Part model, mm, in its own coordinate system. A direction names the side the tool comes from. Coordinates: 2 decimals unless noted, no trailing zeros. Order: outer loops, then holes, each group sorted by start corner. A loop starts at its lowest first (then second) coordinate and runs counter-clockwise, first axis right, second up. Notation, with made-up numbers: (18, 46.5) - (70, 46.5) arc R18 ccw to (70, 55.5) - close; hole circle Ø5 at (50, 44). An arc over 180 degrees is marked (long way). Use a Markdown table: item, result. Add a question column.
1) Two-plate mould, pull along X, no slides. Class faces 1 (the face through (6, 14, 51)), 2 (the face through (11, 5.8, 44)), 3 (the face through (11, 16.3, 44)), 4 (the face through (10, 5, 0)): +X half, -X half, draft (parallel to the pull), parting line (faces both ways), or undercut.
2) Tool access for faces 5 (the face through (11, 20, 80)), 6 (the face through (7, 8.3, 44)), 7 (the face through (10, 17, 0)), 8 (the face through (15, 6, 44)): list every direction of +Z, -Z, +X, -X, +Y, -Y with a clear straight run to the whole face (end or side of a thin tool).
3) Saw through at B-B on x = 14. List the corners of the cut face in (y, z), then the cut area to 3 significant figures.
4) Wall check: L1, parallel to Y at x = 8.75, z = 13; L2, parallel to Y at x = 11.25, z = 56; L3, parallel to Z at x = 15, y = 9.25. Give the ranges that are in metal, low to high. Write a range as [from, to].
5) Saw through at A-A on z = 31. List the corners of the cut face in (x, y).
6) Drop flat-ended pins along their axis: P1, Ø1.1, axis at x = 14, z = 64.5, coming from the +Y side; P2, Ø1.3, axis at y = 7, z = 53, coming from the +X side; P3, Ø3, axis at x = 14, y = 11, coming from the -Z side; P4, Ø1, axis at y = 11.5, z = 22, coming from the -X side. Give the stop position or say it passes through.
7) Saw through at D-D on x = 10. List the corners of the cut face in (y, z), then the cut area to 3 significant figures.
8) Saw through at C-C on y = 19.75. List the corners of the cut face in (x, z), then the cut area to 3 significant figures.
```python
from build123d import *

# Parameters (mm, degrees)
SKETCH2_W           = 3.75
SKETCH2_H           = 0.3
SKETCH2_H_2         = 0.2
BOSS_EXTRUDE3_DEPTH = 90
SKETCH3_W           = 10.75
SKETCH3_H           = 15.726491146
BOSS_EXTRUDE4_DEPTH = 10
SKETCH4_W           = 10.75
SKETCH4_H           = 2.578461227
BOSS_EXTRUDE5_DEPTH = 20


with BuildPart() as part:
    # Sketch2 → Boss-Extrude3 (new body)
    with BuildSketch(Plane.XY):
        with Locations((14.875, 16.15)):
            Rectangle(SKETCH2_W, SKETCH2_H)
        Polygon((8.7, 16.3), (8.7, 18.913245573), (16.75, 18.913245573), (16.75, 16.3), (13, 16.3), align=None)
        Polygon((6, 18.913245573), (6, 13.8), (8.7, 13.8), (8.7, 16.3), (8.7, 18.913245573), align=None)
        Polygon((8.8, 3.186754427), (8.8, 5.8), (8.8, 8.3), (6, 8.3), (6, 3.186754427), align=None)
        Polygon((8.8, 5.8), (13, 5.8), (16.75, 5.8), (16.75, 3.186754427), (8.8, 3.186754427), align=None)
        with Locations((14.875, 5.9)):
            Rectangle(SKETCH2_W, SKETCH2_H_2)
    extrude(amount=BOSS_EXTRUDE3_DEPTH)

    # Sketch3 → Boss-Extrude4 (add)
    with BuildSketch(Plane.XY.offset(90)):
        with Locations((11.375, 11.05)):
            Rectangle(SKETCH3_W, SKETCH3_H)
    extrude(amount=BOSS_EXTRUDE4_DEPTH)

    # Sketch4 → Boss-Extrude5 (add)
    with BuildSketch(Plane.XY.offset(100)):
        with Locations((11.375, 20.202476187)):
            Rectangle(SKETCH4_W, SKETCH4_H)
    extrude(amount=-BOSS_EXTRUDE5_DEPTH)


solid = part.part
```
Results are:
| question | item | result |
|---|---|---|
| 1 | face 1 | -X half |
| 1 | face 2 | undercut |
| 1 | face 3 | undercut |
| 1 | face 4 | draft |
| 2 | face 5 | -Z, +X, -X, +Y |
| 2 | face 6 | -Z, +X, -X |
| 2 | face 7 | -Z, +X, -X, +Y, -Y |
| 2 | face 8 | -Z, +X |
| 3 | outline | (3.19, 0) - (6, 0) - (6, 90) - (16, 90) - (16, 0) - (18.91, 0) - (18.91, 80) - (21.49, 80) - (21.49, 100) - (3.19, 100) - close |
| 3 | area | 724 mm2 |
| 4 | L1 | [3.19, 8.3], [16.3, 18.91] |
| 4 | L2 | [3.19, 5.8], [16.3, 18.91] |
| 4 | L3 | [90, 100] |
| 5 | outline | (6, 3.19) - (16.75, 3.19) - (16.75, 6) - (13, 6) - (13, 5.8) - (8.8, 5.8) - (8.8, 8.3) - (6, 8.3) - close; (6, 13.8) - (8.7, 13.8) - (8.7, 16.3) - (13, 16.3) - (13, 16) - (16.75, 16) - (16.75, 18.91) - (6, 18.91) - close |
| 6 | P1 | y = 18.91 |
| 6 | P2 | x = 8.8 |
| 6 | P3 | z = 90 |
| 6 | P4 | through |
| 7 | outline | (3.19, 0) - (5.8, 0) - (5.8, 90) - (16.3, 90) - (16.3, 0) - (18.91, 0) - (18.91, 80) - (21.49, 80) - (21.49, 100) - (3.19, 100) - close |
| 7 | area | 679 mm2 |
| 8 | outline | (6, 80) - (16.75, 80) - (16.75, 100) - (6, 100) - close |
| 8 | area | 215 mm2 |
